Check sheet for the modelled part. Datum: model origin and axes. Units: mm. Face numbers are marked on the shaded views. A direction names the side the tool comes from. Give positions to 0.01 mm unless a question says otherwise; leave off trailing zeros. Order: outer loops, then holes, each group sorted by start corner. A loop starts at its lowest first (then second) coordinate and runs counter-clockwise, first axis right, second up.
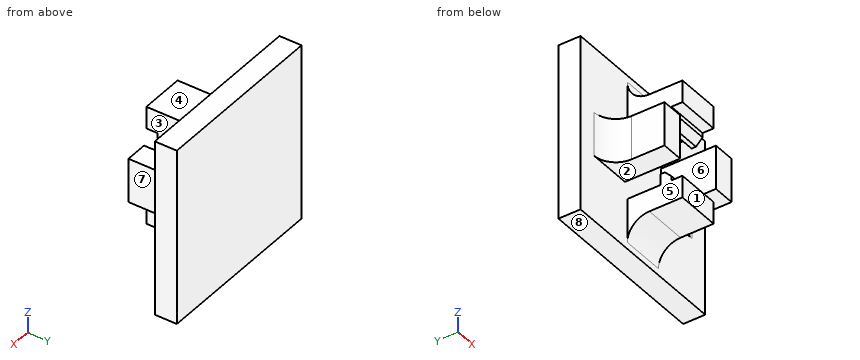
from build123d import *

# Parameters (mm, degrees)
SKETCH1_W                = 8
SKETCH1_H                = 8
BOSS_EXTRUDE1_DEPTH      = 1
SKETCH2_W                = 2
SKETCH2_H                = 1
SKETCH2_W_2              = 1
SKETCH2_H_2              = 2
BOSS_EXTRUDE2_DEPTH      = 2.5
SKETCH3_W                = 2
SKETCH3_H                = 0.5
BOSS_EXTRUDE3_DEPTH      = 0.5
CHAMFER2_SIZE            = 0.3
CHAMFER2_OF_MIRROR2_SIZE = 0.3
FILLET1_R                = 1


with BuildPart() as part:
    # Sketch1 → Boss-Extrude1 (new body)
    with BuildSketch(Plane(origin=(0, 0, 0), x_dir=(1, 0, 0), z_dir=(0, 1, 0))):
        Rectangle(SKETCH1_W, SKETCH1_H)
    extrude(amount=BOSS_EXTRUDE1_DEPTH)

    # Sketch2 → Boss-Extrude2 (add)
    with BuildSketch(Plane.XZ):
        with Locations((0, 2.2)):
            Rectangle(SKETCH2_W, SKETCH2_H)
        with Locations((1.65, 0)):
            Rectangle(SKETCH2_W_2, SKETCH2_H_2)
    boss_extrude2 = extrude(amount=BOSS_EXTRUDE2_DEPTH)

    # Sketch3 → Boss-Extrude3 (add)
    with BuildSketch(Plane(origin=(0, 0, 1.7), x_dir=(-1, 0, 0), z_dir=(0, 0, -1))):
        with Locations((0, -1.75)):
            Rectangle(SKETCH3_W, SKETCH3_H)
    boss_extrude3 = extrude(amount=BOSS_EXTRUDE3_DEPTH)

    # Chamfer2
    chamfer2_edges = [part.edges().sort_by_distance(p)[0] for p in [
        (0, -2, 1.2),
    ]]
    chamfer(chamfer2_edges, length=CHAMFER2_SIZE)

    # Mirror1: Boss-Extrude2 across plane
    add(boss_extrude2.mirror(Plane(origin=(0, 0, 0), x_dir=(0, 0, 1), z_dir=(1, 0, 0))))

    # Mirror2: Boss-Extrude2, Boss-Extrude3 across plane
    add(boss_extrude2.mirror(Plane.XY))
    add(boss_extrude3.mirror(Plane.XY))

    # Chamfer2 of Mirror2
    chamfer2_of_mirror2_edges = [part.edges().sort_by_distance(p)[0] for p in [
        (0, -2, -1.2),
    ]]
    chamfer(chamfer2_of_mirror2_edges, length=CHAMFER2_OF_MIRROR2_SIZE)

    # Fillet1
    fillet1_edges = [part.edges().sort_by_distance(p)[0] for p in [
        (0, 0, 2.7),
        (2.15, 0, 0),
        (-2.15, 0, 0),
        (0, 0, -2.7),
    ]]
    fillet(fillet1_edges, radius=FILLET1_R)


solid = part.part
1) Draft check along X on the marked faces 6, 7 and 8. Enter one of: +X half, -X half, draft (parallel to the pull), parting line (faces both ways), or undercut.
Recorded:
face 6: undercut
face 7: +X half
face 8: draft
2) Section check D-D, the plane y = -0.75. Record the cut outline in (x, z), then the cut area to 3 significant figures.
Recorded:
outline: (-2.18, -1) - (-1.15, -1) - (-1.15, 1) - (-2.18, 1) - close; (-1, -2.73) - (1, -2.73) - (1, -1.7) - (-1, -1.7) - close; (-1, 1.7) - (1, 1.7) - (1, 2.73) - (-1, 2.73) - close; (1.15, -1) - (2.18, -1) - (2.18, 1) - (1.15, 1) - close
area: 8.25 mm2
3) Section check C-C, the plane z = 0.25. Record the cut outline in (x, y).
Recorded:
outline: (-4, 0) - (-3.15, 0) arc R1 cw to (-2.15, -1) - (-2.15, -2.5) - (-1.15, -2.5) - (-1.15, 0) - (1.15, 0) - (1.15, -2.5) - (2.15, -2.5) - (2.15, -1) arc R1 cw to (3.15, 0) - (4, 0) - (4, 1) - (-4, 1) - close
4) Depth check by flat-ended pin: pin 1 Ø0.8 at (x, y) = (0, -1.5) entering from -Z; pin 2 Ø0.8 at (y, z) = (-1.5, -2.5) entering from +X; pin 3 Ø1.2 at (y, z) = (-1, 3) entering from -X. Enter the tip coordinate at first touch or a pass-through.
Recorded:
pin 1: stops at z = -2.7
pin 2: stops at x = 1
pin 3: stops at x = -1
5) Section check B-B, the plane x = -0.5. Record the cut outline in (y, z), then the cut area to 3 significant figures.
Recorded:
outline: (-2.5, -2.7) - (-1, -2.7) arc R1 cw to (0, -3.7) - (0, -4) - (1, -4) - (1, 4) - (0, 4) - (0, 3.7) arc R1 cw to (-1, 2.7) - (-2.5, 2.7) - (-2.5, 1.7) - (-2, 1.7) - (-2, 1.5) - (-1.7, 1.2) - (-1.5, 1.2) - (-1.5, 1.7) - (0, 1.7) - (0, -1.7) - (-1.5, -1.7) - (-1.5, -1.2) - (-1.7, -1.2) - (-2, -1.5) - (-2, -1.7) - (-2.5, -1.7) - close
area: 13.8 mm2
6) Set-up check for the marked faces 1, 2, 3, 4 and 5: record each of +Z, -Z, +X, -X, +Y, -Y from which the full face is reachable in a straight line by a thin tool's end or side.
Recorded:
face 1: +Z, -Z, +X, -X, -Y
face 2: -Z, +X, -X, -Y
face 3: +Z, -Z, +X, -Y
face 4: +Z, +X, -X, -Y
face 5: +Z, -Z, -X, -Y
7) Material ranges on L1, parallel to X at y = -1.8, z = -0.5; L2, parallel to Y at x = 1.75, z = -2.25; L3, parallel to X at y = -1.1, z = 2.5, recorded low to high.
Recorded:
L1: x = -2.15 to -1.15, 1.15 to 2.15
L2: y = 0 to 1
L3: x = -1 to 1
8) Section check A-A, the plane y = -1.8. Record the cut outline in (x, z).
Recorded:
outline: (-2.15, -1) - (-1.15, -1) - (-1.15, 1) - (-2.15, 1) - close; (-1, -2.7) - (1, -2.7) - (1, -1.3) - (-1, -1.3) - close; (-1, 1.3) - (1, 1.3) - (1, 2.7) - (-1, 2.7) - close; (1.15, -1) - (2.15, -1) - (2.15, 1) - (1.15, 1) - close
